Can you work these out from the model? Positions are in its coordinate system, mm. A direction names the side the tool comes from. Round coordinates to 2 decimals unless told otherwise and drop trailing zeros. Order: outer loops, then holes, each group sorted by start corner. A loop starts at its lowest first (then second) coordinate and runs counter-clockwise, first axis right, second up. Notation, with made-up numbers: (7, 67) - (52, 67) arc R12 cw to (52, 86) - close; hole circle Ø7 at (4.5, 66). An arc over 180 degrees is marked (long way). Write item = value, one per line.
from build123d import *

# Parameters (mm, degrees)
F0_W     = 480.568
F0_H     = 139.7
F1_DEPTH = 12.7
F2_R     = 2.54
F3_DEPTH = 25.4
F4_R     = 25.4


with BuildPart() as f1:
    # F0 (on Top) → F1 (new body)
    with BuildSketch(Plane.XY):
        with Locations((192.473375, 50.443076)):
            Rectangle(F0_W, F0_H)
    extrude(amount=-F1_DEPTH)

    # F2 (on face) → F3 (cut)
    with BuildSketch(Plane.XY):
        with Locations((-35.110625, 25.043076)):
            Circle(F2_R)
        with BuildLine():
            Line((271.960707, 91.714286), (112.209601, 91.718076))
            ThreePointArc((112.209601, 91.718076), (102.684375, 82.193076), (112.209601, 72.668076))
            Line((112.209601, 72.668076), (271.960707, 72.671866))
            ThreePointArc((271.960707, 72.671866), (281.754375, 82.193076), (271.960707, 91.714286))
        make_face()
        with Locations((40.073375, 25.043076)):
            Circle(F2_R)
        with Locations((344.873375, 25.043076)):
            Circle(F2_R)
        with Locations((420.057375, 25.043076)):
            Circle(F2_R)
    extrude(amount=-F3_DEPTH, mode=Mode.SUBTRACT)

    # F4
    f4_edges = [f1.edges().sort_by_distance(p)[0] for p in [
        (-47.810625, -19.406924, -6.35),
        (432.757375, -19.406924, -6.35),
    ]]
    fillet(f4_edges, radius=F4_R)


solid = f1.part
(1) If we section it at C-C (x = 255): Write out the boundary of the cut face in (y, z).
Computed:
outline = (-19.41, -12.7) - (72.67, -12.7) - (72.67, 0) - (-19.41, 0) - close; (91.71, -12.7) - (120.29, -12.7) - (120.29, 0) - (91.71, 0) - close
(2) If I drill on line 1 (Y direction, x = 228.5, z = -3.75); line 2 (X direction, y = 81, z = -6); line 3 (Y direction, x = 281, z = -5.75), over which ranges is the centre line in solid material (lowest first)? Write a range as from..to.
Computed:
line_1 = -19.41..72.67, 91.72..120.29
line_2 = -47.81..102.76, 281.68..432.76
line_3 = -19.41..78.48, 85.91..120.29
(3) If we section it at B-B (z = -5.75): Write out the boundary of the cut face in (x, y) (3 decimals), plus the area to 3 significant figures.
Computed:
outline = (-47.811, 5.993) arc R25.4 ccw to (-22.411, -19.407) - (407.357, -19.407) arc R25.4 ccw to (432.757, 5.993) - (432.757, 120.293) - (-47.811, 120.293) - close; hole circle Ø5.08 at (-35.111, 25.043); hole circle Ø5.08 at (40.073, 25.043); hole (112.21, 72.668) - (271.961, 72.672) arc R9.525 ccw (long way) to (271.961, 91.714) - (112.21, 91.718) arc R9.525 ccw to start; hole circle Ø5.08 at (344.873, 25.043); hole circle Ø5.08 at (420.057, 25.043)
area = 63,400 mm^2
(4) If we section it at A-A (x = 176): Write out the boundary of the cut face in (y, z), plus the area to 3 significant figures.
Computed:
outline = (-19.41, -12.7) - (72.67, -12.7) - (72.67, 0) - (-19.41, 0) - close; (91.72, -12.7) - (120.29, -12.7) - (120.29, 0) - (91.72, 0) - close
area = 1,530 mm^2
(5) Will these pins go through, and if not, where does the flat tip stop? P1, Ø3, axis at x = 344.87, y = 25.04, coming from the -Z side; P2, Ø1.5, axis at y = 1.5, z = -11, coming from the +X side.
Computed:
P1 = through
P2 = 432.48
(6) On a 3-axis mill with a long thin cutter (end or side, diameter ignored), from which of +Z, -Z, +X, -X, +Y, -Y can I reach the whole of each face in a straight line? I mean faces 1 (the face through (102.687, 82.403, -6.261)), 2 (the face through (189, 51, -12.7)). Say none if no direction works.
Computed:
face_1 = +Z, -Z
face_2 = -Z, +X, -X, +Y, -Y
(7) Thinking about a two-plate mould opening in Y: for faces 3 (the face through (189, 51, 0)), 4 (the face through (425.119, -12.164, -6.439)), 5 (the face through (281.75, 81.98, -6.26)), which applies, +Y half, -Y half, draft (parallel to the pull), parting line (faces both ways), or undercut?
Computed:
face_3 = draft
face_4 = -Y half
face_5 = undercut
